from build123d import *

# Parameters (mm, degrees)
RESSALTO_EXTRUS_O1_DEPTH = 50
ESBO_O2_W                = 5.2
ESBO_O2_H                = 2.5
ESBO_O2_W_2              = 2.5
ESBO_O2_H_2              = 5.2
CORTE_EXTRUS_O1_DEPTH    = 6
ESBO_O3_R                = 0.5
CORTE_EXTRUS_O2_DEPTH    = 0.4


with BuildPart() as part:
    # Esboço1 → Ressalto-extrusão1 (new body)
    with BuildSketch(Plane.XY):
        Polygon((0, 0), (0, 50), (50, 0), align=None)
    extrude(amount=RESSALTO_EXTRUS_O1_DEPTH)

    # Esboço2 → Corte-extrusão1 (cut)
    with BuildSketch(Plane.XZ):
        with Locations((25, 28.85)):
            Rectangle(ESBO_O2_W, ESBO_O2_H)
        with Locations((21.15, 25)):
            Rectangle(ESBO_O2_W_2, ESBO_O2_H_2)
        with Locations((25, 25)):
            Rectangle(ESBO_O2_W, ESBO_O2_H_2)
        with Locations((28.85, 25)):
            Rectangle(ESBO_O2_W_2, ESBO_O2_H_2)
        with Locations((25, 21.15)):
            Rectangle(ESBO_O2_W, ESBO_O2_H)
    extrude(amount=-CORTE_EXTRUS_O1_DEPTH, mode=Mode.SUBTRACT)

    # Esboço3 → Corte-extrusão2 (cut)
    with BuildSketch(Plane(origin=(25, 25, 0), x_dir=(0, 0, -1), z_dir=(0.7071067811865487, 0.7071067811865465, 0))):
        with Locations(Location((-25, 0, 0), (0, 0, 90))):
            Circle(ESBO_O3_R)
    extrude(amount=-CORTE_EXTRUS_O2_DEPTH, mode=Mode.SUBTRACT)


solid = part.part
CAD build for the part. Positions are in the model's coordinates, mm. A direction names the side the tool comes from. Round coordinates to 2 decimals unless told otherwise and drop trailing zeros. Loops run counter-clockwise (first coordinate to the right, second up) from the corner with the lowest first, then second, coordinate; pieces in that order, holes last. Notation, with made-up numbers: M 38,76 L 60,76 A12 cw 60,91 Z; hole C 2,48 d2. An arc over 180 degrees is marked long. One line per question, with ' | ' between items. Start each with the question number.
Item 1: Wall check: line 1 (Z direction, x = 21.5, y = 5); line 2 (X direction, y = 11, z = 33); line 3 (X direction, y = 48.5, z = 43.5). Give the ranges that are in metal, low to high.
Item 2: Cut at C-C, the plane x = 5.5. Write the cut outline in (y, z), plus the area to 4 significant figures.
Item 3: Which spindle directions (+Z, -Z, +X, -X, +Y, -Y) get a long thin tool onto all of the face, cutting with end or side? Do faces 1 (the flat face through (14, 14, 50)), 2 (the flat face through (27.6, 3, 21)). Say none if no direction does.
Item 4: Two-plate mould, pull along X, no slides. Class faces 3 (the flat face through (14, 14, 0)), 4 (the flat face through (25, 6, 25)), 5 (the flat face through (0, 25, 25)): pulls with the +X half, pulls with the -X half, needs draft (parallel to the pull), parting line crosses it, or undercut.
Item 5: Cut at B-B, the plane z = 29. Write the cut outline in (x, y).
Item 6: Cut at A-A, the plane y = 3.5. Write the cut outline in (x, z).
Item 7: Cut at D-D, the plane y = 21. Write the cut outline in (x, z).
Item 8: Pin check, flat tips, straight feed: pin 1 Ø3 at (y, z) = (4, 22) entering from -X; pin 2 Ø12 at (y, z) = (11.5, 29) entering from +X; pin 3 Ø12 at (x, z) = (41, 25.5) entering from +Y; pin 4 Ø1.2 at (y, z) = (3, 21) entering from +X. Stop position of each tip, or through.
Responses:
1) line 1: z = 0 to 22.4, 27.6 to 50 | line 2: x = 0 to 39 | line 3: x = 0 to 1.5
2) outline: M 0,0 L 44.5,0 L 44.5,50 L 0,50 Z | area: 2,225 mm²
3) face 1: +Z, +X, -X, +Y, -Y | face 2: -Y
4) face 3: needs draft | face 4: undercut | face 5: pulls with the -X half
5) outline: M 0,0 L 22.4,0 L 22.4,6 L 27.6,6 L 27.6,0 L 50,0 L 0,50 Z
6) outline: M 0,0 L 46.5,0 L 46.5,50 L 0,50 Z; hole M 19.9,22.4 L 22.4,22.4 L 22.4,19.9 L 27.6,19.9 L 27.6,22.4 L 30.1,22.4 L 30.1,27.6 L 27.6,27.6 L 27.6,30.1 L 22.4,30.1 L 22.4,27.6 L 19.9,27.6 Z
7) outline: M 0,0 L 29,0 L 29,50 L 0,50 Z
8) pin 1: stops at x = 0 | pin 2: stops at x = 44.5 | pin 3: stops at y = 15 | pin 4: stops at x = 47.6
